from build123d import *

# Parameters (mm, degrees)
BOSS_EXTRUDE1_DEPTH     = 20
FILLET1_R               = 10
SKETCH2_R               = 20
CUT_EXTRUDE1_DEPTH      = 20
TAP_DRILL_FOR_M5_TAP1_D = 4.2
M5_CLEARANCE_HOLE1_D    = 5.5
TAP_DRILL_FOR_M5_TAP2_D = 4.2
FILLET2_R               = 4


with BuildPart() as part:
    # Sketch1 → Boss-Extrude1 (new body)
    with BuildSketch(Plane.XY):
        with BuildLine():
            Line((-170.200000001, 540.824594888), (-129.309401077, 470))
            Line((-129.309401077, 470), (-93, 470))
            ThreePointArc((-93, 470), (-90.878679656, 470.878679656), (-90, 473))
            Line((-90, 473), (-90, 564.25527297))
            Line((-90, 564.25527297), (-116.225329238, 607))
            Line((-116.225329238, 607), (-170.200000001, 607))
            Line((-170.200000001, 607), (-170.200000001, 540.824594888))
        make_face()
    extrude(amount=BOSS_EXTRUDE1_DEPTH)

    # Fillet1
    fillet1_edges = [part.edges().sort_by_distance(p)[0] for p in [
        (-90, 564.25527297, 10),
        (-129.309401077, 470, 10),
        (-170.200000001, 540.824594888, 10),
    ]]
    fillet(fillet1_edges, radius=FILLET1_R)

    # Sketch2 → Cut-Extrude1 (cut)
    with BuildSketch(Plane.XY.offset(20)):
        with Locations((-142.000000001, 577)):
            Circle(SKETCH2_R)
    extrude(amount=-CUT_EXTRUDE1_DEPTH, mode=Mode.SUBTRACT)

    # Tap Drill for M5 Tap1 (through all)
    with Locations(Plane(origin=(0, 0, 0), x_dir=(-1, 0, 0), z_dir=(0, 0, -1))):
        with Locations((160.000000001, 600), (142.000000001, 600), (142.000000001, 554), (160.000000001, 554)):
            Hole(TAP_DRILL_FOR_M5_TAP1_D / 2)

    # M5 Clearance Hole1 (through all)
    with Locations(Plane.XY.offset(20)):
        with Locations((-95, 545), (-125, 545), (-125, 475), (-95, 475), (-110, 490), (-110, 530)):
            Hole(M5_CLEARANCE_HOLE1_D / 2)

    # Tap Drill for M5 Tap2 (through all)
    with Locations(Plane.XY.offset(20)):
        with Locations((-165.570000001, 553.43), (-165.570000001, 600.57), (-118.430000001, 553.43), (-118.430000001, 600.57)):
            Hole(TAP_DRILL_FOR_M5_TAP2_D / 2)

    # Fillet2
    fillet2_edges = [part.edges().sort_by_distance(p)[0] for p in [
        (-116.225329238, 607, 10),
        (-170.200000001, 607, 10),
    ]]
    fillet(fillet2_edges, radius=FILLET2_R)


solid = part.part
Can you work these out from the model? Positions are in its coordinate system, mm. Give positions to 0.01 mm unless a question says otherwise; leave off trailing zeros. Loops run counter-clockwise (first coordinate to the right, second up) from the corner with the lowest first, then second, coordinate; pieces in that order, holes last. Notation, with made-up numbers: M -28,29 L 23,29 A14 cw 23,36 Z; hole C 53,-5 d5. An arc over 180 degrees is marked long. One line per item, written item: value. Start each with the question number.
1) If we section it at B-B, the plane y = 530: Write out the boundary of the cut face in (x, z).
2) If we section it at D-D, the plane x = -110: Write out the boundary of the cut face in (y, z).
3) Thinking about a two-plate mould opening in X: for faces 1 (the face through (-124.642, 477.727, 9.86)), 2 (the face through (-169.85, 540.88, 10.14)), 3 (the face through (-122, 539, 20)), which applies, +X half, -X half, draft (parallel to the pull), parting line (faces both ways), or undercut?
4) If I drill on line 1 (X direction, y = 545, z = 9.5); line 2 (Y direction, x = -118.43, z = 15); line 3 (Y direction, x = -125.5, z = 13.25), over which ranges is the centre line in solid material (lowest first)? Write a range as [from, to].
5) If we section it at C-C, the plane x = -160: Write out the boundary of the cut face in (y, z).
6) If we section it at A-A, the plane z = 4.25: Give the number of separate pieces and of enclosed holes in the cut face, and give its area (3 significant figures).
7) I'm going to push flat-ended pins straight in: pin 1 (1.5 mm diameter, centred on x = -126, z = 11.5, fed in from -Y); pin 2 (8 mm diameter, centred on x = -162, z = 16.5, fed in from -Y). Where does each tip first touch, or does it pass through?
Completed:
1. outline: M -163.95,0 L -112.75,0 L -112.75,20 L -163.95,20 Z; M -107.25,0 L -90,0 L -90,20 L -107.25,20 Z
2. outline: M 470,0 L 487.25,0 L 487.25,20 L 470,20 Z; M 492.75,0 L 527.25,0 L 527.25,20 L 492.75,20 Z; M 532.75,0 L 596.85,0 L 596.85,20 L 532.75,20 Z
3. face 1: undercut
3. face 2: -X half
3. face 3: draft
4. line 1: x = [-170.2, -127.75], [-122.25, -97.75], [-92.25, -90]
4. line 2: y = [470, 551.33], [555.53, 598.47], [602.67, 607]
4. line 3: y = [470.19, 472.3], [477.7, 542.3], [547.7, 565.7], [588.3, 607]
5. outline: M 523.16,0 L 551.9,0 L 551.9,20 L 523.16,20 Z; M 556.1,0 L 568.28,0 L 568.28,20 L 556.1,20 Z; M 585.72,0 L 597.9,0 L 597.9,20 L 585.72,20 Z; M 602.1,0 L 607,0 L 607,20 L 602.1,20 Z
6. separate pieces: 1
6. enclosed holes: 15
6. area: 7,460 mm^2
7. pin 1: stops at y = 470.15
7. pin 2: stops at y = 519.69
